Source: CAD feature listing. Evaluate the final solid. Frame: model axes, mm. A direction names the side the tool comes from. Round coordinates to 2 decimals unless told otherwise and drop trailing zeros. Loops run counter-clockwise (first coordinate to the right, second up) from the corner with the lowest first, then second, coordinate; pieces in that order, holes last. Notation, with made-up numbers: M 42,6.25 L 89,6.25 A24 cw 89,22.25 Z; hole C 68.25,-19.75 d7. An arc over 180 degrees is marked long. Answer as a JSON object with one key per item and string values.
from build123d import *

# Parameters (mm, degrees)
CROQUIS1_W              = 45.25
CROQUIS1_H              = 20.4
CROQUIS1_R              = 8
SALIENTE_EXTRUIR1_DEPTH = 2
CROQUIS2_R              = 8
SALIENTE_EXTRUIR2_DEPTH = 13.8
CROQUIS3_W              = 10.45
CROQUIS3_H              = 2.5
SALIENTE_EXTRUIR4_DEPTH = 4.3
CROQUIS4_W              = 10.45
CROQUIS4_H              = 2
SALIENTE_EXTRUIR5_DEPTH = 6.4


with BuildPart() as part:
    # Croquis1 → Saliente-Extruir1 (new body)
    with BuildSketch(Plane(origin=(0, 0, 0), x_dir=(1, 0, 0), z_dir=(0, 1, 0))):
        with Locations((1.264210019, -2.135211946)):
            Rectangle(CROQUIS1_W, CROQUIS1_H)
        with Locations(Location((-10.222061657, -2.135211946, 0), (0, 0, 270))):
            Circle(CROQUIS1_R, mode=Mode.SUBTRACT)
        with Locations(Location((12.749210019, -2.135211946, 0), (0, 0, 270))):
            Circle(CROQUIS1_R, mode=Mode.SUBTRACT)
    extrude(amount=SALIENTE_EXTRUIR1_DEPTH)

    # Croquis2 → Saliente-Extruir2 (add)
    with BuildSketch(Plane(origin=(0, 0, 0), x_dir=(-1, 0, 0), z_dir=(0, -1, 0))):
        with Locations(Location((10.222061657, -2.135211946, 0), (0, 0, 90))):
            Circle(CROQUIS2_R)
        with Locations(Location((-12.749210019, -2.135211946, 0), (0, 0, 90))):
            Circle(CROQUIS2_R)
    extrude(amount=-SALIENTE_EXTRUIR2_DEPTH)

    # Croquis3 → Saliente-Extruir4 (add)
    with BuildSketch(Plane(origin=(0, 0, 0), x_dir=(-1, 0, 0), z_dir=(0, -1, 0))):
        with Locations((-1.264210019, 6.814788054)):
            Rectangle(CROQUIS3_W, CROQUIS3_H)
    extrude(amount=SALIENTE_EXTRUIR4_DEPTH)

    # Croquis4 → Saliente-Extruir5 (add)
    with BuildSketch(Plane(origin=(0, 0, -8.064788054), x_dir=(-1, 0, 0), z_dir=(0, 0, -1))):
        with Locations((-1.264210019, -3.3)):
            Rectangle(CROQUIS4_W, CROQUIS4_H)
    extrude(amount=SALIENTE_EXTRUIR5_DEPTH)


solid = part.part
Item 1: Contact query for flat-ended pins moving along their axis: pin 1 Ø4.5 at (x, y) = (1, 0) entering from -Z; pin 2 Ø7 at (x, z) = (2, -12) entering from +Y; pin 3 Ø2 at (x, z) = (8.5, 0) entering from -Y; pin 4 Ø1.5 at (x, z) = (-6, -11) entering from -Y. Output: stop coordinate, or through.
Answer sheet:
{"pin 1": "stops at z = -8.06", "pin 2": "stops at y = -2.3", "pin 3": "stops at y = 0", "pin 4": "passes through"}
Item 2: Access query for faces 5 (the flat face through (6.489, -3, -9)), 6 (the flat face through (1, -3, -14.465)), 7 (the flat face through (1, -2.3, -11)), 8 (the flat face through (1, 2, 2)), 9 (the flat face through (1, -2, -5.565)). Directions: +Z, -Z, +X, -X, +Y, -Y. A direction counts if a zero-diameter tool reaches every point of the face in a straight line with its end or side. Return the directions, or none.
Answer sheet:
{"face 5": "+Z, -Z, +X, -Y", "face 6": "-Z, +X, -X, +Y, -Y", "face 7": "-Z, +X, -X, +Y", "face 8": "+Y", "face 9": "+Z, +X, -X, -Y"}
Item 3: Section C-C on y = 0.5. Return the cut outline in (x, z).
Answer sheet:
{"outline": "M -21.36,-8.06 L 23.89,-8.06 L 23.89,12.34 L -21.36,12.34 Z"}
Item 4: Pull-direction query (X, two-part tool) for faces 1 (the cylindrical face through (9.685, 7.817, -5.255)), 2 (the cylindrical face through (-2.29, 7.82, 3.18)), 3 (the flat face through (-3.961, -3, -9)), 4 (the flat face through (1, 1, -8.065)); classes: pulls with the +X half, pulls with the -X half, needs draft (parallel to the pull), parting line crosses it, or undercut.
Answer sheet:
{"face 1": "undercut", "face 2": "undercut", "face 3": "pulls with the -X half", "face 4": "needs draft"}
Item 5: Line query: probe 1 along X at (y, z) = (13.25, 2); probe 2 along Y at (x, z) = (-6, -5.25); probe 3 along Z at (x, y) = (4.5, -3.5). Output: solid intervals per line, ascending. Write a range as from..to.
Answer sheet:
{"probe 1": "x = -18.22..-2.22, 4.75..20.75", "probe 2": "y = 0..2", "probe 3": "z = -14.46..-5.56"}
Item 6: Section B-B on z = -4.25. Return the cut outline in (x, y), then the cut area to 3 significant figures.
Answer sheet:
{"outline": "M -21.36,0 L 23.89,0 L 23.89,2 L 17.57,2 L 17.57,13.8 L 7.93,13.8 L 7.93,2 L -5.4,2 L -5.4,13.8 L -15.04,13.8 L -15.04,2 L -21.36,2 Z", "area": "318 mm²"}
Item 7: Section D-D on y = 9.5. Return the cut outline in (x, z).
Answer sheet:
{"outline": "C -10.22,2.14 d16; C 12.75,2.14 d16"}
Item 8: Section A-A on x = 1.5. Return the cut outline in (y, z).
Answer sheet:
{"outline": "M -4.3,-14.46 L -2.3,-14.46 L -2.3,-8.06 L 2,-8.06 L 2,12.34 L 0,12.34 L 0,-5.56 L -4.3,-5.56 Z"}
